from build123d import *

# Parameters (mm, degrees)
BASE_FLANGE1_DEPTH  = 2.5
SKETCH6_W           = 6
SKETCH6_H           = 3.5
CUT_EXTRUDE1_DEPTH  = 10
SKETCH7_W           = 10
SKETCH7_H           = 2.5
BOSS_EXTRUDE1_DEPTH = 10


# Sheet-metal steps are written as plain solids
with BuildPart() as part:
    # Sketch1 → Base-Flange1 (new body)
    with BuildSketch(Plane.XY):
        Polygon((-35, 0), (35, 0), (8.412017167, 33), (5, 33), (5, 43), (-5, 43), (-5, 33), (-8.412017167, 33), align=None)
    extrude(amount=-BASE_FLANGE1_DEPTH)

    # Sketch6 → Cut-Extrude1 (cut)
    with BuildSketch(Plane.XY):
        with Locations((0, 38)):
            Rectangle(SKETCH6_W, SKETCH6_H)
    extrude(amount=-CUT_EXTRUDE1_DEPTH, mode=Mode.SUBTRACT)

    # Sketch7 → Boss-Extrude1 (add)
    with BuildSketch(Plane.XY):
        with Locations((-27.985758876, 1.25)):
            Rectangle(SKETCH7_W, SKETCH7_H)
    boss_extrude1 = extrude(amount=BOSS_EXTRUDE1_DEPTH)

    # Mirror1: Boss-Extrude1 across plane
    add(boss_extrude1.mirror(Plane(origin=(0, 0, 0), x_dir=(0, 0, 1), z_dir=(1, 0, 0))))


solid = part.part
Input: part model. Units: mm. Frame: model coordinates. A direction names the side the tool comes from. Give positions to 0.01 mm unless a question says otherwise; leave off trailing zeros. Order: outer loops, then holes, each group sorted by start corner. A loop starts at its lowest first (then second) coordinate and runs counter-clockwise, first axis right, second up. Notation, with made-up numbers: (68.5, 39) - (96.5, 39) arc R13 ccw to (96.5, 45) - close; hole circle Ø9 at (37, -37). An arc over 180 degrees is marked (long way). Answer as a JSON object with one key per item and string values. Group by question number.
Q1. Mould query, pull axis X, two halves, no side actions, for faces 1 (the face through (-7, 33, -1)), 2 (the face through (22.986, 1, 5)), 3 (the face through (32.986, 1, 5)), 4 (the face through (-5, 38, -1)). Classes: pulls with the +X half, pulls with the -X half, needs draft (parallel to the pull), parting line crosses it, or undercut.
Q2. Line query: probe 1 along X at (y, z) = (2, 8.25); probe 2 along Z at (x, y) = (-21, 13); probe 3 along Y at (x, z) = (26, 8.5). Output: solid intervals per line, ascending.
Q3. Cut plane B-B, the plane x = 2. Output: boundary loops of the cut face in (y, z), then the cut area to 4 significant figures.
Q4. First-contact query: pin 1 Ø3 at (x, z) = (-7.5, -1) entering from +Y; pin 2 Ø3 at (y, z) = (18.5, 0) entering from +X; pin 3 Ø0.8 at (y, z) = (37.5, -1) entering from -X. Flat tips, straight axial feed; report the tip coordinate or a pass-through.
Q5. Cut plane D-D, the plane x = -25.5. Output: boundary loops of the cut face in (y, z), then the cut area to 3 significant figures.
Q6. Cut plane A-A, the plane z = 8. Output: boundary loops of the cut face in (x, y), then the cut area to 3 significant figures.
Q7. Set-up query: faces 5 (the face through (0, 36.25, -1)), 6 (the face through (-34, 1, 0)), 7 (the face through (5, 38, -1)), 8 (the face through (-28, 2.5, 5)). Return all of +Z, -Z, +X, -X, +Y, -Y with unobstructed straight access to the full face (end or side cutting, diameter ignored); none if empty.
Q8. Cut plane C-C, the plane y = 22. Output: boundary loops of the cut face in (x, z).
Results:
{
 "1": {"face 1": "needs draft", "face 2": "undercut", "face 3": "pulls with the +X half", "face 4": "pulls with the -X half"},
 "2": {"probe 1": "-32.99 to -22.99, 22.99 to 32.99", "probe 2": "-2.5 to 0", "probe 3": "0 to 2.5"},
 "3": {"outline": "(0, -2.5) - (36.25, -2.5) - (36.25, 0) - (0, 0) - close; (39.75, -2.5) - (43, -2.5) - (43, 0) - (39.75, 0) - close", "area": "98.75 mm^2"},
 "4": {"pin 1": "y = 33", "pin 2": "x = 21.3", "pin 3": "x = -5"},
 "5": {"outline": "(0, -2.5) - (11.79, -2.5) - (11.79, 0) - (2.5, 0) - (2.5, 10) - (0, 10) - close", "area": "54.5 mm^2"},
 "6": {"outline": "(-32.99, 0) - (-22.99, 0) - (-22.99, 2.5) - (-32.99, 2.5) - close; (22.99, 0) - (32.99, 0) - (32.99, 2.5) - (22.99, 2.5) - close", "area": "50.0 mm^2"},
 "7": {"face 5": "+Z, -Z", "face 6": "+Z, -X, +Y, -Y", "face 7": "+Z, -Z, +X, +Y", "face 8": "+Z, +X, -X, +Y"},
 "8": {"outline": "(-17.27, -2.5) - (17.27, -2.5) - (17.27, 0) - (-17.27, 0) - close"}
}
